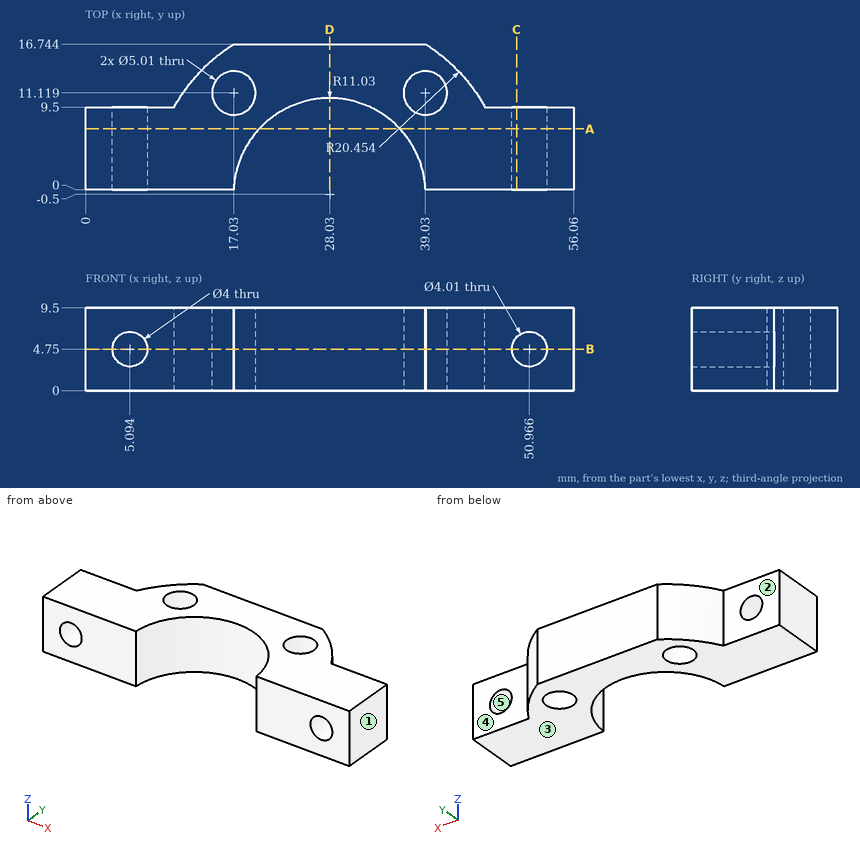
Input: dimensioned drawing with shaded views. Units: mm. Origin: part minimum x, y, z. A direction names the side the tool comes from. Coordinates: 2 decimals unless noted, no trailing zeros. Loops run counter-clockwise (first coordinate to the right, second up) from the corner with the lowest first, then second, coordinate; pieces in that order, holes last. Notation, with made-up numbers: (65, -24) -> (113, -24) arc R22 cw to (113, 1) -> close; hole circle Ø9 at (42, -22.5). An arc over 180 degrees is marked (long way). Use a Markdown table: item, result. Add a question column.
(1) Mould query, pull axis Z, two halves, no side actions, for the marked faces 3, 4 and 5. Classes: pulls with the +Z half, pulls with the -Z half, needs draft (parallel to the pull), parting line crosses it, or undercut.
(2) Line query: line 1 along X through (y, z) = (4.5, 5.25) (1 decimal); line 2 along X through (y, z) = (9, 3.5) (1 decimal); line 3 along X through (y, z) = (1.25, 3) (1 decimal). Output: solid intervals per line, ascending.
(3) Section query A-A, the plane y = 7. State how many separate pieces and enclosed holes the cut face has, plus the area to 3 significant figures.
(4) Section query B-B, the plane z = 4.75. Return loops of the section in (x, y) (1 decimal), plus the area to 3 significant figures.
(5) Access query for the marked faces 1 and 2. Directions: +Z, -Z, +X, -X, +Y, -Y. A direction counts if a zero-diameter tool reaches every point of the face in a straight line with its end or side. Return the directions, or none.
(6) Section query D-D, the plane x = 28.03. Return loops of the section in (y, z) (1 decimal).
(7) Section query C-C, the plane x = 49.5. Return loops of the section in (y, z).
(8) Pin query (flat end, axial travel): pin 1 Ø5 at (x, z) = (51, 3.5) entering from +Y; pin 2 Ø3 at (x, z) = (5.09, 4.75) entering from +Y; pin 3 Ø1 at (x, z) = (12.5, 2) entering from +Y (1 decimal). Return the tip coordinate at first contact, or that it passes through.
Answer:
| question | item | result |
|---|---|---|
| 1 | face 3 | pulls with the -Z half |
| 1 | face 4 | needs draft |
| 1 | face 5 | undercut |
| 2 | line 1 | x = 0 to 3.2, 7 to 18.2, 37.9 to 49, 52.9 to 56.1 |
| 2 | line 2 | x = 0 to 3.5, 6.7 to 15.7, 18.4 to 22.4, 33.6 to 37.7, 40.4 to 49.4, 52.5 to 56.1 |
| 2 | line 3 | x = 0 to 4.1, 6.1 to 17.1, 38.9 to 50, 51.9 to 56.1 |
| 3 | separate pieces | 2 |
| 3 | enclosed holes | 2 |
| 3 | area | 354 mm^2 |
| 4 | outline | (0, 0) -> (3.1, 0) -> (3.1, 9.5) -> (0, 9.5) -> close; (7.1, 0) -> (17, 0) arc R11 cw to (39, 0) -> (49, 0) -> (49, 9.5) -> (45.9, 9.5) arc R20.5 ccw to (39, 16.7) -> (17, 16.7) arc R20.5 ccw to (10.2, 9.5) -> (7.1, 9.5) -> close; (53, 0) -> (56.1, 0) -> (56.1, 9.5) -> (53, 9.5) -> close; hole circle Ø5 at (17, 11.1); hole circle Ø5 at (39, 11.1) |
| 4 | area | 454 mm^2 |
| 5 | face 1 | +Z, -Z, +X, +Y, -Y |
| 5 | face 2 | +Z, -Z, -X, +Y |
| 6 | outline | (10.5, 0) -> (16.7, 0) -> (16.7, 9.5) -> (10.5, 9.5) -> close |
| 7 | outline | (0, 0) -> (9.5, 0) -> (9.5, 3.38) -> (0, 3.38) -> close; (0, 6.12) -> (9.5, 6.12) -> (9.5, 9.5) -> (0, 9.5) -> close |
| 8 | pin 1 | stops at y = 9.5 |
| 8 | pin 2 | passes through |
| 8 | pin 3 | stops at y = 13.4 |
